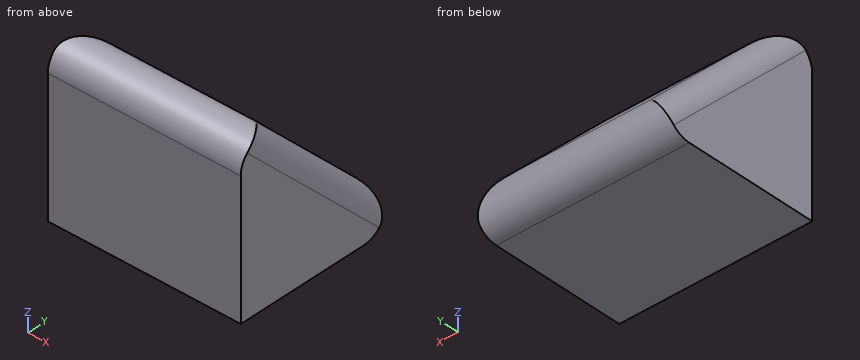
```python
from build123d import *

# Parameters (mm, degrees)
F1_DEPTH = 8
F2_R     = 1


with BuildPart() as f1:
    # F0 (on Right) → F1 (new body)
    with BuildSketch(Plane.YZ):
        Polygon((0, 8), (0, 0), (8, 0), align=None)
    extrude(amount=F1_DEPTH)

    # F2
    f2_edges = [f1.edges().sort_by_distance(p)[0] for p in [
        (4, 0, 8),
        (4, 8, 0),
        (0, 4, 4),
        (8, 4, 4),
    ]]
    fillet(f2_edges, radius=F2_R)


solid = f1.part
```
For this review, take the finished solid that the model builds, in its own axes (mm). Round coordinates to 2 decimals unless told otherwise and drop trailing zeros. Write each loop counter-clockwise with the first axis right and the second up, starting at its lowest first coordinate (ties: lowest second). Pieces come first, ordered by that corner, then holes. Notation, with made-up numbers: M -22.75,82 L 11.25,82 A19 cw 11.25,117 Z; hole C 55.25,75 d3. An arc over 180 degrees is marked long. One line per item, written item: value. Start each with the question number.
(1) Wall thickness on line 1 (Z direction, x = 4.5, y = 5.75); line 2 (Y direction, x = 6.25, z = 2.5); line 3 (Z direction, x = 7.5, y = 1.5): over which ranges is each line inside the solid? List them lowest first.
(2) Insertion check: pin 1 (2 mm diameter, centred on x = 3.5, y = 5.5, fed in from +Z); pin 2 (1.5 mm diameter, centred on x = 1, z = 3, fed in from +Y). Each pin has a flat end and moves straight along its axis. Give the tip position at first contact, or say it passes through.
(3) We need section A-A (x = 4.25). Give the boundary of the cut face in (y, z).
Result:
1. line 1: 0.01 to 2.25
1. line 2: 0 to 5.5
1. line 3: 0 to 6.31
2. pin 1: z = 3.5
2. pin 2: y = 5.75
3. outline: M 0,0 L 5.59,0 A1 ccw 6.29,1.71 L 1.71,6.29 A1 ccw 0,5.59 Z
